The listing builds one solid part. Answer for the finished solid, in the listing's coordinates (mm). Face numbers are marked on the shaded views. A direction names the side the tool comes from. Coordinates: 2 decimals unless noted, no trailing zeros. Loops run counter-clockwise (first coordinate to the right, second up) from the corner with the lowest first, then second, coordinate; pieces in that order, holes last. Notation, with made-up numbers: (27, 53.25) - (46, 53.25) arc R30 ccw to (46, 77.25) - close; hole circle Ø1 at (-25.75, 70.25). An arc over 180 degrees is marked (long way). One line per question, with ' | ' between items.
from build123d import *

# Parameters (mm, degrees)
SKETCH140_R          = 2.75
SKETCH140_R_2        = 1.3208
SKETCH140_W          = 6
SKETCH140_H          = 8
PAD083_DEPTH         = 20
POCKET048_DEPTH      = 14
SKETCH160_W          = 20
SKETCH160_H          = 20
POCKET059_DEPTH      = 25.001
POCKET059_DEPTH_BACK = 25.001


with BuildPart() as part:
    # Sketch140 → Pad083 (new body)
    with BuildSketch(Plane.XY):
        with BuildLine():
            Line((-28.743574, 9.167173), (-10, 25))
            Line((-10, 25), (10, 25))
            Line((10, 25), (10, -25))
            Line((10, -25), (-10, -25))
            Line((-10, -25), (-24, -25))
            ThreePointArc((-26.88165, -22.83432), (-25.802365, -24.398224), (-24, -25))
            Line((-32.526602, -3.337282), (-26.88165, -22.83432))
            ThreePointArc((-28.743574, 9.167173), (-32.485873, 3.474872), (-32.526602, -3.337282))
        make_face()
        with Locations((0, 15)):
            Circle(SKETCH140_R, mode=Mode.SUBTRACT)
        with Locations((0, -15)):
            Circle(SKETCH140_R, mode=Mode.SUBTRACT)
        with Locations((-21, -10)):
            Circle(SKETCH140_R_2, mode=Mode.SUBTRACT)
        with Locations((-21, -18)):
            Rectangle(SKETCH140_W, SKETCH140_H, mode=Mode.SUBTRACT)
    extrude(amount=PAD083_DEPTH)

    # Sketch141 → Pocket048 (cut)
    with BuildSketch(Plane.XY):
        with BuildLine():
            Line((-17.75, -8.660254), (-17.75, -22))
            Line((-17.75, -22), (-24.25, -22))
            Line((-24.25, -22), (-24.25, -8.660254))
            ThreePointArc((-17.75, -8.660254), (-21, 9.25), (-24.25, -8.660254))
        make_face()
    extrude(amount=POCKET048_DEPTH, mode=Mode.SUBTRACT)

    # Sketch160 → Pocket059 (cut, two sides)
    with BuildSketch(Plane.XZ) as pocket059_sk:
        with Locations((0, 22)):
            Rectangle(SKETCH160_W, SKETCH160_H)
    extrude(amount=-POCKET059_DEPTH, mode=Mode.SUBTRACT)
    extrude(pocket059_sk.sketch, amount=POCKET059_DEPTH_BACK, mode=Mode.SUBTRACT)


solid = part.part
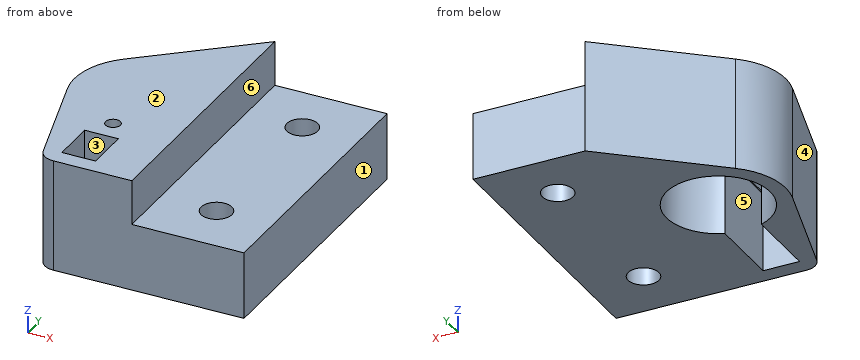
Item 1: Which of the six approach directions +Z, -Z, +X, -X, +Y, -Y give full straight-line access (tool end or side, diameter ignored) to the marked faces 4, 5 and 6?
Taken from the geometry:
face 4: +Z, -Z, -X, -Y | face 5: -Z | face 6: +Z, +X, +Y, -Y
Item 2: Find section A-A, the plane x = 0. Write down the section's boundary in (y, z).
Taken from the geometry:
outline: (-25, 0) - (-17.75, 0) - (-17.75, 12) - (-25, 12) - close; (-12.25, 0) - (12.25, 0) - (12.25, 12) - (-12.25, 12) - close; (17.75, 0) - (25, 0) - (25, 12) - (17.75, 12) - close
Item 3: Find section B-B, the plane z = 2. Write down the section's boundary in (x, y).
Taken from the geometry:
outline: (-32.53, -3.34) - (-26.88, -22.83) arc R3 ccw to (-24, -25) - (10, -25) - (10, 25) - (-10, 25) - (-28.74, 9.17) arc R12 ccw to start; hole (-24.25, -22) - (-17.75, -22) - (-17.75, -8.66) arc R9.25 ccw (long way) to (-24.25, -8.66) - close; hole circle Ø5.5 at (0, -15); hole circle Ø5.5 at (0, 15)
Item 4: Each of these flat-tipped pins is pushed along its axis until it touches: pin 1 Ø10.5 at (y, z) = (-16.5, 5.5) entering from -X; pin 2 Ø12 at (y, z) = (8.5, 4.5) entering from -X; pin 3 Ø1 at (x, y) = (4, -9.5) entering from +Z. Where does it stop, or does it pass through?
Taken from the geometry:
pin 1: stops at x = -30.24 | pin 2: stops at x = -32.74 | pin 3: stops at z = 12
Item 5: Find section C-C, the plane y = -10. Write down the section's boundary in (x, z), plus the area to 3 significant figures.
Taken from the geometry:
outline: (-30.6, 0) - (-24.25, 0) - (-24.25, 14) - (-22.32, 14) - (-22.32, 20) - (-30.6, 20) - close; (-19.68, 14) - (-17.75, 14) - (-17.75, 0) - (10, 0) - (10, 12) - (-10, 12) - (-10, 20) - (-19.68, 20) - close | area: 545 mm2
Item 6: Find the intervals of material crossed by line 1 (Y direction, x = 0, z = 8); line 2 (X direction, y = 0, z = 9.25); line 3 (X direction, y = -14.5, z = 2.75), in increasing order. Write a range as [from, to].
Taken from the geometry:
line 1: y = [-25, -17.75], [-12.25, 12.25], [17.75, 25] | line 2: x = [-33, -30.25], [-11.75, 10] | line 3: x = [-29.29, -24.25], [-17.75, -2.7], [2.7, 10]
Item 7: Find section D-D, the plane y = 0. Write down the section's boundary in (x, z), plus the area to 3 significant figures.
Taken from the geometry:
outline: (-33, 0) - (-30.25, 0) - (-30.25, 14) - (-11.75, 14) - (-11.75, 0) - (10, 0) - (10, 12) - (-10, 12) - (-10, 20) - (-33, 20) - close | area: 441 mm2
Item 8: The mould has two halves that part along X. Classify the marked faces 1, 2 and 3: pulls with the +X half, pulls with the -X half, needs draft (parallel to the pull), parting line crosses it, or undercut.
Taken from the geometry:
face 1: pulls with the +X half | face 2: needs draft | face 3: undercut
